Geometry check sheet. Reference: the model listing, model coordinates, mm. A direction names the side the tool comes from. Round coordinates to 2 decimals unless told otherwise and drop trailing zeros. Write each loop counter-clockwise with the first axis right and the second up, starting at its lowest first coordinate (ties: lowest second). Pieces come first, ordered by that corner, then holes. Notation, with made-up numbers: (86.5, 59.25) -> (124.5, 59.25) arc R23 cw to (124.5, 83.25) -> close; hole circle Ø6 at (16, 69). An arc over 180 degrees is marked (long way). Use a Markdown table: item, result.
```python
from build123d import *

# Parameters (mm, degrees)
SKETCH_2_R          = 12
EXTRUDE_1_DEPTH     = 30
SKETCH_3_R          = 18
EXTRUDE_2_DEPTH     = 45
SKETCH_4_R          = 16
CUT_EXTRUDE_1_DEPTH = 43
FILLET_1_R          = 2


with BuildPart() as part:
    # 草图1 → 旋转1 (revolve)
    with BuildSketch(Plane.XY, mode=Mode.PRIVATE) as revolve_1_sk:
        Polygon((0, 20), (-4, 20), (-4, 19), (-15, 19), (-15, 0), (0, 0), align=None)
    revolve_1 = revolve(revolve_1_sk.sketch.rotate(Axis((0, 20, 0), (0, -1, 0)), 270), axis=Axis((0, 20, 0), (0, -1, 0)))

    # 镜向1: 旋转1 across plane
    add(revolve_1.mirror(Plane(origin=(0, 0, 0), x_dir=(0, 0, 1), z_dir=(0, -1, 0))))

    # 草图2 → 凸台-拉伸1 (add)
    with BuildSketch(Plane(origin=(0, 0, 0), x_dir=(0, 0, -1), z_dir=(1, 0, 0))):
        with Locations(Location((0, 0, 0), (0, 0, 180))):
            Circle(SKETCH_2_R)
    extrude(amount=EXTRUDE_1_DEPTH)

    # 草图3 → 凸台-拉伸2 (add)
    with BuildSketch(Plane(origin=(30, 0, 0), x_dir=(0, 0, -1), z_dir=(1, 0, 0))):
        with Locations(Location((0, 0, 0), (0, 0, 180))):
            Circle(SKETCH_3_R)
    extrude(amount=EXTRUDE_2_DEPTH)

    # 草图4 → 切除-拉伸1 (cut)
    with BuildSketch(Plane(origin=(75, 0, 0), x_dir=(0, 0, -1), z_dir=(1, 0, 0))):
        Circle(SKETCH_4_R)
    extrude(amount=-CUT_EXTRUDE_1_DEPTH, mode=Mode.SUBTRACT)

    # 圆角1
    fillet_1_edges = [part.edges().sort_by_distance(p)[0] for p in [
        (30, 0, -18),
        (75, 0, -18),
    ]]
    fillet(fillet_1_edges, radius=FILLET_1_R - 0.0001)  # a hair under: the kernel refuses the full size


solid = part.part
```
(1) Section check C-C on x = 43. Record the cut outline in (y, z), plus the area to 3 significant figures.
A:
| item | result |
|---|---|
| outline | circle Ø36 at (0, 0); hole circle Ø32 at (0, 0) |
| area | 214 mm2 |
(2) Thickness scan on line 1 (Y direction, x = 64.5, z = 0); line 2 (Y direction, x = -6.5, z = -0.5); line 3 (Z direction, x = 65, y = -1). Record the ranges inside material, lowest first.
A:
| item | result |
|---|---|
| line 1 | y = -18 to -16, 16 to 18 |
| line 2 | y = -19 to 19 |
| line 3 | z = -17.97 to -15.97, 15.97 to 17.97 |
(3) Access from +Z, -Z, +X, -X, +Y, -Y to the whole of each face (thin tool, end or side, straight path). Record for faces 1 (the face through (3, -19, -3)), 2 (the face through (3.905, 19.493, -0.867)), 3 (the face through (21.686, -8.11, -8.844)).
A:
| item | result |
|---|---|
| face 1 | -Y |
| face 2 | +Y |
| face 3 | none |
(4) Section check A-A on x = 0. Record the cut outline in (y, z), plus the area to 3 significant figures.
A:
| item | result |
|---|---|
| outline | (-20, -4) -> (-19, -4) -> (-19, -15) -> (19, -15) -> (19, -4) -> (20, -4) -> (20, 4) -> (19, 4) -> (19, 15) -> (-19, 15) -> (-19, 4) -> (-20, 4) -> close |
| area | 1,160 mm2 |
(5) Release check for a two-part mould opening along Z. For faces 4 (the face through (30, -12, 2)), 5 (the face through (32, 0, 0)), 6 (the face through (53.8, -15.62, 3.47)), 7 (the face through (3.905, -19.493, -0.867)) record: +Z half, -Z half, draft (parallel to the pull), parting line (faces both ways), or undercut.
A:
| item | result |
|---|---|
| face 4 | draft |
| face 5 | undercut |
| face 6 | undercut |
| face 7 | parting line |
(6) Section check D-D on x = 12.5. Record the cut outline in (y, z), plus the area to 3 significant figures.
A:
| item | result |
|---|---|
| outline | (-19, -8.29) -> (-8.67, -8.29) arc R12 ccw to (8.67, -8.29) -> (19, -8.29) -> (19, 8.29) -> (8.67, 8.29) arc R12 ccw to (-8.67, 8.29) -> (-19, 8.29) -> close |
| area | 719 mm2 |
(7) Gauge pin test, flat ends, axial feed: pin 1 Ø3 at (x, y) = (25.5, -4.5) entering from -Z; pin 2 Ø10 at (x, z) = (26.5, -10) entering from -Y; pin 3 Ø2 at (y, z) = (8, -11) entering from +X; pin 4 Ø2 at (x, z) = (25.5, 13.5) entering from +Y. Record the tip position at first contact, or that the pin passes through.
A:
| item | result |
|---|---|
| pin 1 | stops at z = -11.62 |
| pin 2 | stops at y = -15.95 |
| pin 3 | stops at x = 32 |
| pin 4 | passes through |
